from build123d import *

# Parameters (mm, degrees)
CROQUIS1_W              = 25
CROQUIS1_H              = 25
SALIENTE_EXTRUIR1_DEPTH = 50
CORTAR_EXTRUIR1_DEPTH   = 6


with BuildPart() as part:
    # Croquis1 → Saliente-Extruir1 (new body)
    with BuildSketch(Plane.XY):
        with Locations((12.5, 12.5)):
            Rectangle(CROQUIS1_W, CROQUIS1_H)
    extrude(amount=SALIENTE_EXTRUIR1_DEPTH)

    # Croquis2 → Cortar-Extruir1 (cut)
    with BuildSketch(Plane.XY.offset(50)):
        Polygon((18.273502692, 12.5), (15.386751346, 17.5), (9.613248654, 17.5), (6.726497308, 12.5), (9.613248654, 7.5), (15.386751346, 7.5), align=None)
    extrude(amount=-CORTAR_EXTRUIR1_DEPTH, mode=Mode.SUBTRACT)


solid = part.part
Input: part model. Units: mm. Frame: model coordinates. A direction names the side the tool comes from. Give positions to 0.01 mm unless a question says otherwise; leave off trailing zeros. Loops run counter-clockwise (first coordinate to the right, second up) from the corner with the lowest first, then second, coordinate; pieces in that order, holes last. Notation, with made-up numbers: M 64.5,25 L 98.5,25 A3 ccw 98.5,29 Z; hole C 39.5,18.25 d10. An arc over 180 degrees is marked long. Use one line per item in the form item = value.
1. Line query: L1, parallel to Y at x = 8, z = 47; L2, parallel to X at y = 10.75, z = 47; L3, parallel to Z at x = 15, y = 13.25. Output: solid intervals per line, ascending.
Numbers:
L1 = 0 to 10.29, 14.71 to 25
L2 = 0 to 7.74, 17.26 to 25
L3 = 0 to 44
2. First-contact query: pin 1 (3 mm diameter, centred on x = 14.5, y = 13.5, fed in from +Z). Flat tip, straight axial feed; report the tip coordinate or a pass-through.
Numbers:
pin_1 = 44
3. Section query A-A, the plane x = 13.75. Return the cut outline in (y, z), and give its area (3 significant figures).
Numbers:
outline = M 0,0 L 25,0 L 25,50 L 17.5,50 L 17.5,44 L 7.5,44 L 7.5,50 L 0,50 Z
area = 1,190 mm²
4. Section query B-B, the plane y = 16.75. Return the cut outline in (x, z).
Numbers:
outline = M 0,0 L 25,0 L 25,50 L 15.82,50 L 15.82,44 L 9.18,44 L 9.18,50 L 0,50 Z
5. Pull-direction query (X, two-part tool) for faces 3 (the face through (0, 12, 25)), 4 (the face through (12, 0, 25)), 5 (the face through (25, 12, 25)), 6 (the face through (13, 17.5, 47)); classes: released by +X, released by -X, zero draft, split by the parting line, or undercut.
Numbers:
face_3 = released by -X
face_4 = zero draft
face_5 = released by +X
face_6 = undercut
6. Reachability of faces 1 (the face through (16.85, 14.965, 47.042)), 2 (the face through (12, 7, 50)) from +Z, -Z, +X, -X, +Y, -Y: full face, straight path, thin tool, end or side. Return the list, or none.
Numbers:
face_1 = +Z
face_2 = +Z, +X, -X, +Y, -Y
